Input: dimensioned drawing with shaded views. Units: mm. Origin: part minimum x, y, z. A direction names the side the tool comes from. Round coordinates to 2 decimals unless told otherwise and drop trailing zeros. Write each loop counter-clockwise with the first axis right and the second up, starting at its lowest first coordinate (ties: lowest second). Pieces come first, ordered by that corner, then holes. Notation, with made-up numbers: (67.5, 13) -> (92.5, 13) arc R26 cw to (92.5, 45) -> close; hole circle Ø1 at (41.5, -1.5). An arc over 180 degrees is marked (long way). Use one line per item in the form item = value. Start each with the question number.
1. Reachability of the marked faces 4 and 5 from +Z, -Z, +X, -X, +Y, -Y: full face, straight path, thin tool, end or side. Return the list, or none.
2. Draft query along X for the marked faces 1, 2 and 3. Return one class per face: pulls with the +X half, pulls with the -X half, needs draft (parallel to the pull), parting line crosses it, or undercut.
3. Cut plane B-B, the plane y = 2.25. Return the cut outline in (x, z) (1 decimal).
4. Cut plane C-C, the plane z = 3. Return the cut outline in (x, y) (1 decimal).
5. Line query: L1, parallel to Y at x = 11.25, z = 3.25 (1 decimal); L2, parallel to X at y = 10.25, z = 1.25 (1 decimal); L3, parallel to Z at x = 11, y = 8.5. Output: solid intervals per line, ascending.
6. Cut plane A-A, the plane x = 11. Return the cut outline in (y, z) (1 decimal).
7. Pin query (flat end, axial travel): pin 1 Ø1.5 at (y, z) = (3, 3) entering from -X; pin 2 Ø1 at (x, y) = (12, 5) entering from -Z; pin 3 Ø2 at (y, z) = (6, 3) entering from -X. Return the tip coordinate at first contact, or that it passes through.
8. Cut plane D-D, the plane x = 3.5. Return the cut outline in (y, z) (1 decimal).
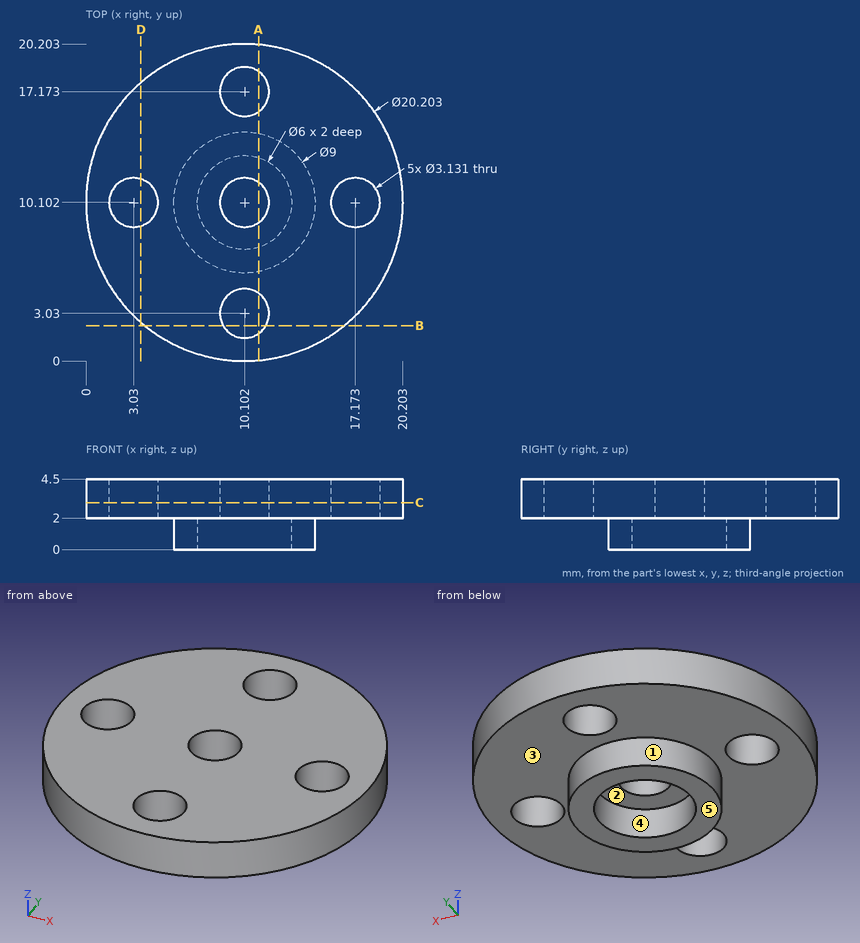
Outcome:
q1.face_4 = -Z
q1.face_5 = -Z, +X, -X, +Y, -Y
q2.face_1 = parting line crosses it
q2.face_2 = undercut
q2.face_3 = needs draft
q3.outline = (3.7, 2) -> (8.7, 2) -> (8.7, 4.5) -> (3.7, 4.5) -> close; (11.5, 2) -> (16.5, 2) -> (16.5, 4.5) -> (11.5, 4.5) -> close
q4.outline = circle Ø20.2 at (10.1, 10.1); hole circle Ø3.1 at (3, 10.1); hole circle Ø3.1 at (10.1, 3); hole circle Ø3.1 at (10.1, 10.1); hole circle Ø3.1 at (10.1, 17.2); hole circle Ø3.1 at (17.2, 10.1)
q5.L1 = 0.1 to 2, 4.1 to 9, 11.2 to 16.1, 18.2 to 20.1
q5.L2 = 5.6 to 7.1, 13.1 to 14.6
q5.L3 = 2 to 4.5
q6.outline = (0, 2) -> (1.7, 2) -> (1.7, 4.5) -> (0, 4.5) -> close; (4.3, 2) -> (5.7, 2) -> (5.7, 0) -> (7.2, 0) -> (7.2, 2) -> (8.8, 2) -> (8.8, 4.5) -> (4.3, 4.5) -> close; (11.4, 2) -> (13, 2) -> (13, 0) -> (14.5, 0) -> (14.5, 2) -> (15.9, 2) -> (15.9, 4.5) -> (11.4, 4.5) -> close; (18.5, 2) -> (20.2, 2) -> (20.2, 4.5) -> (18.5, 4.5) -> close
q7.pin_1 = 2.25
q7.pin_2 = 2
q7.pin_3 = 0.49
q8.outline = (2.5, 2) -> (8.6, 2) -> (8.6, 4.5) -> (2.5, 4.5) -> close; (11.6, 2) -> (17.7, 2) -> (17.7, 4.5) -> (11.6, 4.5) -> close
